Geometry check sheet. Reference: the model listing, model coordinates, mm. Round coordinates to 2 decimals unless told otherwise and drop trailing zeros. Loops run counter-clockwise (first coordinate to the right, second up) from the corner with the lowest first, then second, coordinate; pieces in that order, holes last. Notation, with made-up numbers: (-33, -19.5) - (-28, -19.5) arc R20 ccw to (-28, 15.5) - close; hole circle Ø1 at (23.5, -3.75). An arc over 180 degrees is marked (long way). Answer as CSV lines item,"result". Start each with the question number.
1) Thickness scan on line 1 along X through (y, z) = (2.5, 101.6); line 2 along X through (y, z) = (3.25, 60); line 3 along Z through (x, y) = (50.8, 2.75). Record the ranges inside material, lowest first.
2) Cross-section at B-B on x = -21.5. Record the boundary of the cut face in (y, z), and give its area (3 significant figures).
3) Cross-section at D-D on x = 50.8. Record the boundary of the cut face in (y, z), and give its area (3 significant figures).
4) Cross-section at C-C on z = -6.35. Record the boundary of the cut face in (x, y), and give its area (3 significant figures).
5) Draft check along Z on faces 1 (the flat face through (-101.6, 3, 47)), 2 (the cylindrical face through (54.214, 3.131, 96.246)), 3 (the cylindrical face through (76.249, 3.131, -87.567)). Enter one of: released by +Z, released by -Z, zero draft, split by the parting line, or undercut.
6) Cross-section at A-A on z = 101.6. Record the boundary of the cut face in (x, y), and give its area (3 significant figures).
from build123d import *

# Parameters (mm, degrees)
SKETCH1_R           = 85.09
SKETCH1_R_2         = 6.35
BOSS_EXTRUDE1_DEPTH = 6.35


with BuildPart() as part:
    # Sketch1 → Boss-Extrude1 (new body)
    with BuildSketch(Plane(origin=(0, 0, 0), x_dir=(1, 0, 0), z_dir=(0, 1, 0))):
        with BuildLine():
            Line((12.7, 114.3), (0, 114.3))
            ThreePointArc((0, 114.3), (-69.761055355, 86.634356609), (-101.6, 18.676470588))
            Line((-101.6, 18.676470588), (-101.6, -114.3))
            Line((-101.6, -114.3), (101.6, -114.3))
            Line((101.6, -114.3), (101.6, 25.4))
            ThreePointArc((101.6, 25.4), (75.561792847, 88.261792847), (12.7, 114.3))
        make_face()
        with Locations((0, 6.35)):
            Circle(SKETCH1_R, mode=Mode.SUBTRACT)
        with Locations((-90.060644326, -24.660366712)):
            Circle(SKETCH1_R_2, mode=Mode.SUBTRACT)
        with Locations((-50.8, -101.6)):
            Circle(SKETCH1_R_2, mode=Mode.SUBTRACT)
        with Locations((50.8, -101.6)):
            Circle(SKETCH1_R_2, mode=Mode.SUBTRACT)
        with Locations((18.17455681, 99.849989223)):
            Circle(SKETCH1_R_2, mode=Mode.SUBTRACT)
        with Locations((71.886087516, -56.139622511)):
            Circle(SKETCH1_R_2, mode=Mode.SUBTRACT)
    extrude(amount=BOSS_EXTRUDE1_DEPTH)


solid = part.part
Answer block:
1,line 1,"x = -101.6 to -57.15, -44.45 to 44.45, 57.15 to 101.6"
1,line 2,"x = -101.6 to -53.27, 53.27 to 66.84, 76.93 to 101.6"
1,line 3,"z = -105.72 to -74.61, 61.91 to 95.25, 107.95 to 114.3"
2,outline,"(0, -112) - (6.35, -112) - (6.35, -88.68) - (0, -88.68) - close; (0, 75.98) - (6.35, 75.98) - (6.35, 114.3) - (0, 114.3) - close"
2,area,"391 mm^2"
3,outline,"(0, -105.72) - (6.35, -105.72) - (6.35, -74.61) - (0, -74.61) - close; (0, 61.91) - (6.35, 61.91) - (6.35, 95.25) - (0, 95.25) - close; (0, 107.95) - (6.35, 107.95) - (6.35, 114.3) - (0, 114.3) - close"
3,area,"450 mm^2"
4,outline,"(-101.6, 0) - (-85.09, 0) - (-85.09, 6.35) - (-101.6, 6.35) - close; (85.09, 0) - (101.6, 0) - (101.6, 6.35) - (85.09, 6.35) - close"
4,area,"210 mm^2"
5,face 1,"zero draft"
5,face 2,"undercut"
5,face 3,"released by -Z"
6,outline,"(-101.6, 0) - (-57.15, 0) - (-57.15, 6.35) - (-101.6, 6.35) - close; (-44.45, 0) - (44.45, 0) - (44.45, 6.35) - (-44.45, 6.35) - close; (57.15, 0) - (101.6, 0) - (101.6, 6.35) - (57.15, 6.35) - close"
6,area,"1,130 mm^2"
